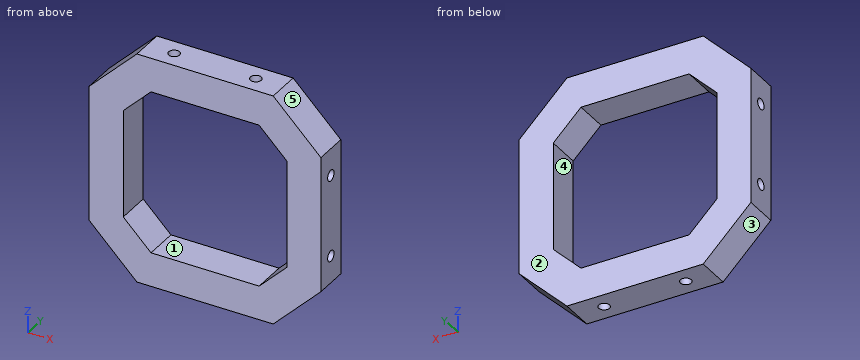
from build123d import *

# Parameters (mm, degrees)
EXTRUDE_1_DEPTH     = 5
SKETCH_2_R          = 0.8
CUT_EXTRUDE_1_DEPTH = 3
CUT_EXTRUDE_START   = -31
SKETCH_2_3_R        = 0.8
CUT_EXTRUDE_2_DEPTH = 3
SKETCH_3_R          = 0.8
CUT_EXTRUDE_3_DEPTH = 3
SKETCH_3_2_R        = 0.8
CUT_EXTRUDE_4_DEPTH = 3


with BuildPart() as part:
    # 草图1 → 凸台-拉伸1 (new body)
    with BuildSketch(Plane(origin=(0, 0, 0), x_dir=(1, 0, 0), z_dir=(0, 1, 0))):
        Polygon((-17, 10), (-17, -10), (-10, -17), (10, -17), (17, -10), (17, 10), (10, 17), (-10, 17), align=None)
        Polygon((-7.928932188, 12), (-12, 7.928932188), (-12, -7.928932188), (-7.928932188, -12), (7.928932188, -12), (12, -7.928932188), (12, 7.928932188), (7.928932188, 12), align=None, mode=Mode.SUBTRACT)
    extrude(amount=EXTRUDE_1_DEPTH)

    # 草图2 → 切除-拉伸1 (cut)
    with BuildSketch(Plane(origin=(0, 0, -17), x_dir=(-1, 0, 0), z_dir=(0, 0, -1))):
        with Locations((6, 2.5)):
            Circle(SKETCH_2_R)
        with Locations((-6, 2.5)):
            Circle(SKETCH_2_R)
    extrude(amount=-CUT_EXTRUDE_1_DEPTH, mode=Mode.SUBTRACT)

    # 草图2<3> → 切除-拉伸2 (cut)
    with BuildSketch(Plane(origin=(0, 0, -17), x_dir=(-1, 0, 0), z_dir=(0, 0, -1)).offset(CUT_EXTRUDE_START)):
        with Locations((6, 2.5)):
            Circle(SKETCH_2_3_R)
        with Locations((-6, 2.5)):
            Circle(SKETCH_2_3_R)
    extrude(amount=-CUT_EXTRUDE_2_DEPTH, mode=Mode.SUBTRACT)

    # 草图3 → 切除-拉伸3 (cut)
    with BuildSketch(Plane.ZY.offset(17)):
        with Locations((-6, 2.5)):
            Circle(SKETCH_3_R)
        with Locations((6, 2.5)):
            Circle(SKETCH_3_R)
    extrude(amount=-CUT_EXTRUDE_3_DEPTH, mode=Mode.SUBTRACT)

    # 草图3<2> → 切除-拉伸4 (cut)
    with BuildSketch(Plane.ZY.offset(17).offset(CUT_EXTRUDE_START)):
        with Locations((-6, 2.5)):
            Circle(SKETCH_3_2_R)
        with Locations((6, 2.5)):
            Circle(SKETCH_3_2_R)
    extrude(amount=-CUT_EXTRUDE_4_DEPTH, mode=Mode.SUBTRACT)


solid = part.part
Check sheet for the modelled part. Datum: model origin and axes. Units: mm. Face numbers are marked on the shaded views. A direction names the side the tool comes from. Round coordinates to 2 decimals unless told otherwise and drop trailing zeros. Loops run counter-clockwise (first coordinate to the right, second up) from the corner with the lowest first, then second, coordinate; pieces in that order, holes last.
1. Set-up check for the marked faces 4 and 5: record each of +Z, -Z, +X, -X, +Y, -Y from which the full face is reachable in a straight line by a thin tool's end or side.
2. Sectioned sample at D-D on z = -1. Record the boundary of the cut face in (x, y).
3. Sectioned sample at C-C on y = 4.35. Record the boundary of the cut face in (x, z).
4. Scan lines: probe 1 along Z at (x, y) = (2, 2.4); probe 2 along Y at (x, z) = (-15.45, 6). Record each from-to range of solid material in increasing order.
5. Sectioned sample at B-B on x = 6. Record the boundary of the cut face in (y, z), and give its area (3 significant figures).
6. Gauge pin test, flat ends, axial feed: pin 1 Ø1.4 at (x, y) = (-6, 2.5) entering from +Z; pin 2 Ø4 at (x, z) = (-9.5, -7.5) entering from +Y; pin 3 Ø0.8 at (x, y) = (-6, 2.5) entering from -Z; pin 4 Ø1 at (y, z) = (2.5, 6) entering from -X. Record the tip position at first contact, or that the pin passes through.
7. Sectioned sample at A-A on z = -6. Record the boundary of the cut face in (x, y).
8. Mould release check, pull along Z, two halves, no side actions. Record for the marked faces 1, 2 and 3: released by +Z, released by -Z, zero draft, split by the parting line, or undercut.
Recorded:
1. face 4: +Y, -Y
1. face 5: +Z, +X, +Y, -Y
2. outline: (-17, 0) - (-12, 0) - (-12, 5) - (-17, 5) - close; (12, 0) - (17, 0) - (17, 5) - (12, 5) - close
3. outline: (-17, -10) - (-10, -17) - (10, -17) - (17, -10) - (17, 10) - (10, 17) - (-10, 17) - (-17, 10) - close; hole (-12, -7.93) - (-7.93, -12) - (7.93, -12) - (12, -7.93) - (12, 7.93) - (7.93, 12) - (-7.93, 12) - (-12, 7.93) - close
4. probe 1: z = -17 to -12, 12 to 17
4. probe 2: y = 0 to 1.7, 3.3 to 5
5. outline: (0, -17) - (1.7, -17) - (1.7, -14) - (3.3, -14) - (3.3, -17) - (5, -17) - (5, -12) - (0, -12) - close; (0, 12) - (5, 12) - (5, 17) - (3.3, 17) - (3.3, 14) - (1.7, 14) - (1.7, 17) - (0, 17) - close
5. area: 40.4 mm2
6. pin 1: stops at z = 14
6. pin 2: passes through
6. pin 3: stops at z = -14
6. pin 4: stops at x = -14
7. outline: (-17, 0) - (-12, 0) - (-12, 5) - (-17, 5) - (-17, 3.3) - (-14, 3.3) - (-14, 1.7) - (-17, 1.7) - close; (12, 0) - (17, 0) - (17, 1.7) - (14, 1.7) - (14, 3.3) - (17, 3.3) - (17, 5) - (12, 5) - close
8. face 1: undercut
8. face 2: zero draft
8. face 3: released by -Z
